The model under review builds one solid part; all positions refer to its coordinate system, in mm. Give positions to 0.01 mm unless a question says otherwise; leave off trailing zeros. Loops run counter-clockwise (first coordinate to the right, second up) from the corner with the lowest first, then second, coordinate; pieces in that order, holes last. Notation, with made-up numbers: (41.25, 31) - (66.25, 31) arc R19 cw to (66.25, 36) - close; hole circle Ø9 at (47, -0.5). An arc over 180 degrees is marked (long way). Return JSON: item names as keys, results as strings. Group by question number.
from build123d import *

# Parameters (mm, degrees)
SKETCH1_R           = 39.6748
SKETCH1_R_2         = 38.1
BOSS_EXTRUDE1_DEPTH = 198.12
SKETCH2_W           = 3.3655
SKETCH2_H           = 121.92
CUT_EXTRUDE1_DEPTH  = 40.6748
CIRPATTERN2_COUNT   = 2
CIRPATTERN2_ANGLE   = 90


with BuildPart() as part:
    # Sketch1 → Boss-Extrude1 (new body, symmetric)
    with BuildSketch(Plane(origin=(0, 0, 0), x_dir=(1, 0, 0), z_dir=(0, 1, 0))):
        Circle(SKETCH1_R)
        Circle(SKETCH1_R_2, mode=Mode.SUBTRACT)
    extrude(amount=BOSS_EXTRUDE1_DEPTH, both=True)

    # Sketch2 → Cut-Extrude1 (cut, symmetric)
    with BuildSketch(Plane(origin=(0, 0, 0), x_dir=(0, 0, -1), z_dir=(1, 0, 0))):
        with Locations((0, -106.68)):
            Rectangle(SKETCH2_W, SKETCH2_H)
    cut_extrude1 = extrude(amount=CUT_EXTRUDE1_DEPTH, both=True, mode=Mode.SUBTRACT)

    # CirPattern2: Cut-Extrude1 ×2 about axis
    cirpattern2_axis = Axis((0, 198.12, 0), (0, -1, 0))
    for i in range(1, CIRPATTERN2_COUNT):
        add(cut_extrude1.rotate(cirpattern2_axis, i * CIRPATTERN2_ANGLE / (CIRPATTERN2_COUNT - 1)), mode=Mode.SUBTRACT)


solid = part.part
Item 1: Take a section at B-B (x = -28). State the section outline as (y, z) points, then the cut area to 3 significant figures.
Item 2: Take a section at D-D (y = 51). State the section outline as (x, z) points.
Item 3: Take a section at A-A (y = -135). State the section outline as (x, z) points.
Item 4: For P1, Ø2, axis at x = 2, y = 8, coming from the +Z side; P2, Ø4, axis at x = 11.5, y = 100.5, coming from the -Z side; P3, Ø12, axis at x = -24.5, y = -46, coming from the -Z side, all flat-tipped, find the tip position at first contact; note any pin that passes through.
Item 5: Take a section at C-C (z = 5). State the section outline as (x, y) points.
Item 6: Mouldability with a two-part tool opening along Z and no side actions: class faces 1 (the face through (-29.242, 2.774, -26.814)), 2 (the face through (-14.9, -198.12, -35.5)), 3 (the face through (36.34, -2.77, -11.44)) as +Z half, -Z half, draft (parallel to the pull), parting line (faces both ways), or undercut.
Item 7: For L1, parallel to X at y = 63, z = 0; L2, parallel to Z at x = -35, y = 13, list the stretches that pass through material, from the lowest coordinate up. Write a range as from..to.
Check sheet entries:
{
 "1": {"outline": "(-198.12, -28.11) - (198.12, -28.11) - (198.12, -25.84) - (-198.12, -25.84) - close; (-198.12, 25.84) - (198.12, 25.84) - (198.12, 28.11) - (-198.12, 28.11) - close", "area": "1,800 mm^2"},
 "2": {"outline": "circle Ø79.35 at (0, 0); hole circle Ø76.2 at (0, 0)"},
 "3": {"outline": "(-39.64, -1.68) arc R39.67 ccw to (-1.68, -39.64) - (-1.68, -38.06) arc R38.1 cw to (-38.06, -1.68) - close; (-39.64, 1.68) - (-38.06, 1.68) arc R38.1 cw to (-1.68, 38.06) - (-1.68, 39.64) arc R39.67 ccw to start; (1.68, -39.64) arc R39.67 ccw to (39.64, -1.68) - (38.06, -1.68) arc R38.1 cw to (1.68, -38.06) - close; (1.68, 38.06) arc R38.1 cw to (38.06, 1.68) - (39.64, 1.68) arc R39.67 ccw to (1.68, 39.64) - close"},
 "4": {"P1": "stops at z = 39.66", "P2": "stops at z = -38.52", "P3": "stops at z = -35.1"},
 "5": {"outline": "(-39.36, -198.12) - (-37.77, -198.12) - (-37.77, 198.12) - (-39.36, 198.12) - close; (37.77, -198.12) - (39.36, -198.12) - (39.36, 198.12) - (37.77, 198.12) - close"},
 "6": {"face 1": "parting line", "face 2": "draft", "face 3": "undercut"},
 "7": {"L1": "x = -39.67..-38.1, 38.1..39.67", "L2": "z = -18.68..-15.05, 15.05..18.68"}
}
